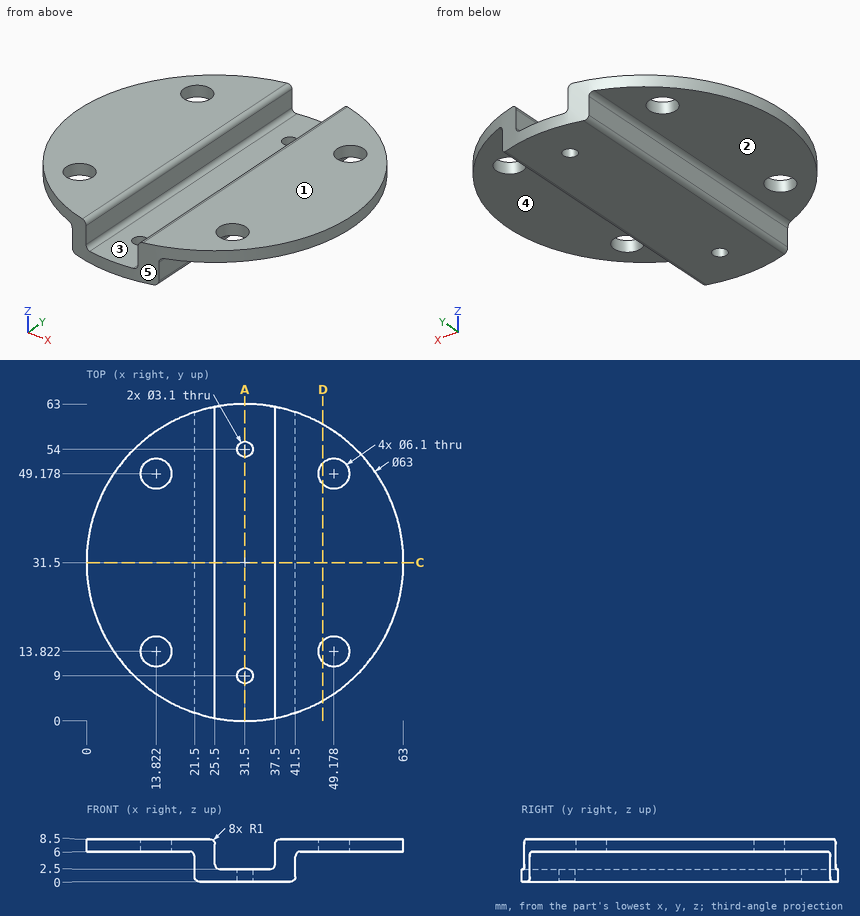
Input: dimensioned drawing with shaded views. Units: mm. Origin: part minimum x, y, z. A direction names the side the tool comes from. Give positions to 0.01 mm unless a question says otherwise; leave off trailing zeros. Loops run counter-clockwise (first coordinate to the right, second up) from the corner with the lowest first, then second, coordinate; pieces in that order, holes last. Notation, with made-up numbers: M -9,75.5 L 50,75.5 A25 ccw 50,89.5 Z; hole C 2,2.25 d9. An arc over 180 degrees is marked long. Put each result on its own line as item: value.
1) Material intervals for L1, parallel to Y at x = 31.5, z = 0.8; L2, parallel to X at y = 9, z = 3.75; L3, parallel to Z at x = 60, y = 29, sorted ascending. Write a range as from..to.
Computed values:
L1: y = 0..7.45, 10.55..52.45, 55.55..63
L2: x = 21.5..25.5, 37.5..41.5
L3: z = 6..8.5
2) Reachability of the marked faces 1 and 2 from +Z, -Z, +X, -X, +Y, -Y: full face, straight path, thin tool, end or side. Return the list, or none.
Computed values:
face 1: +Z, +X, -X, +Y, -Y
face 2: -Z, -X, +Y, -Y
3) Cut plane D-D, the plane x = 47. Return the cut outline in (y, z).
Computed values:
outline: M 4.08,6 L 11.69,6 L 11.69,8.5 L 4.08,8.5 Z; M 15.96,6 L 47.04,6 L 47.04,8.5 L 15.96,8.5 Z; M 51.31,6 L 58.92,6 L 58.92,8.5 L 51.31,8.5 Z
4) Cut plane A-A, the plane x = 31.5. Return the cut outline in (y, z), plus the area to 3 significant figures.
Computed values:
outline: M 0,0 L 7.45,0 L 7.45,2.5 L 0,2.5 Z; M 10.55,0 L 52.45,0 L 52.45,2.5 L 10.55,2.5 Z; M 55.55,0 L 63,0 L 63,2.5 L 55.55,2.5 Z
area: 142 mm^2
5) First-contact query: P1, Ø5, axis at x = 35, z = 2.5, coming from the -Y side; P2, Ø1.9, axis at x = 31.5, y = 54, coming from the +Z side; P3, Ø4, axis at x = 17.5, y = 48.5, coming from the -Z side; P4, Ø3, axis at y = 24.5, z = 2.5, coming from the +X side. Flat tips, straight axial feed; report the tip coordinate or a pass-through.
Computed values:
P1: stops at y = 0.02
P2: passes through
P3: stops at z = 6
P4: stops at x = 41.5
6) Mould query, pull axis X, two halves, no side actions, for the marked faces 3, 4 and 5. Classes: released by +X, released by -X, zero draft, split by the parting line, or undercut.
Computed values:
face 3: undercut
face 4: zero draft
face 5: split by the parting line
7) Cut plane C-C, the plane y = 31.5. Return the cut outline in (x, z).
Computed values:
outline: M 0,6 L 20.5,6 A1 cw 21.5,5 L 21.5,1 A1 ccw 22.5,0 L 40.5,0 A1 ccw 41.5,1 L 41.5,5 A1 cw 42.5,6 L 63,6 L 63,8.5 L 38.5,8.5 A1 ccw 37.5,7.5 L 37.5,3.5 A1 cw 36.5,2.5 L 26.5,2.5 A1 cw 25.5,3.5 L 25.5,7.5 A1 ccw 24.5,8.5 L 0,8.5 Z
